```python
from build123d import *

# Parameters (mm, degrees)
SKETCH2_R           = 25
BOSS_EXTRUDE1_DEPTH = 50
BOSS_EXTRUDE2_DEPTH = 100
CIRPATTERN1_COUNT   = 3
SKETCH5_R           = 150
SKETCH5_R_2         = 90
CUT_EXTRUDE3_DEPTH  = 51
SKETCH3_R           = 6
CUT_EXTRUDE1_DEPTH  = 51


with BuildPart() as part:
    # Sketch2 → Boss-Extrude1 (new body)
    with BuildSketch(Plane(origin=(0, 0, 0), x_dir=(1, 0, 0), z_dir=(0, 1, 0))):
        Circle(SKETCH2_R)
    extrude(amount=BOSS_EXTRUDE1_DEPTH)

    # Sketch4 → Boss-Extrude2 (add)
    with BuildSketch(Plane(origin=(0, 0, 0), x_dir=(0, 0, -1), z_dir=(1, 0, 0))):
        Polygon((10, 50), (8, 50), (-10, 0), (-8, 0), align=None)
    boss_extrude2 = extrude(amount=BOSS_EXTRUDE2_DEPTH)

    # CirPattern1: Boss-Extrude2 ×3 about axis
    cirpattern1_axis = Axis((0, 0, 0), (0, 1, 0))
    for i in range(1, CIRPATTERN1_COUNT):
        add(boss_extrude2.rotate(cirpattern1_axis, i * 360 / CIRPATTERN1_COUNT))

    # Sketch5 → Cut-Extrude3 (cut, through all)
    with BuildSketch(Plane(origin=(0, 50, 0), x_dir=(1, 0, 0), z_dir=(0, 1, 0))):
        Circle(SKETCH5_R)
        Circle(SKETCH5_R_2, mode=Mode.SUBTRACT)
    extrude(amount=-CUT_EXTRUDE3_DEPTH, mode=Mode.SUBTRACT)

    # Sketch3 → Cut-Extrude1 (cut, through all)
    with BuildSketch(Plane(origin=(0, 50, 0), x_dir=(1, 0, 0), z_dir=(0, 1, 0))):
        Circle(SKETCH3_R)
    extrude(amount=-CUT_EXTRUDE1_DEPTH, mode=Mode.SUBTRACT)


solid = part.part
```
Check sheet for the modelled part. Datum: model origin and axes. Units: mm. A direction names the side the tool comes from. Round coordinates to 2 decimals unless told otherwise and drop trailing zeros. Loops run counter-clockwise (first coordinate to the right, second up) from the corner with the lowest first, then second, coordinate; pieces in that order, holes last. Notation, with made-up numbers: (-10, 52) -> (28, 52) arc R31 ccw to (28, 84) -> close; hole circle Ø8 at (19.25, -13). An arc over 180 degrees is marked (long way). Write item = value, one per line. Start each with the question number.
1) Sectioned sample at C-C, the plane y = 31. Record the cut outline in (x, z), plus the area to 3 significant figures.
2) Set-up check for faces 4 (the flat face through (-28.75, 25.35, 48.05)), 5 (the flat face through (-28.75, 24.65, -48.05)), 6 (the cylindrical face through (-45.04, 25.12, 77.92)): record each of +Z, -Z, +X, -X, +Y, -Y from which the full face is reachable in a straight line by a thin tool's end or side.
3) Sectioned sample at B-B, the plane z = 0. Record the cut outline in (x, y).
4) Thickness scan on probe 1 along Z at (x, y) = (0, 29); probe 2 along X at (y, z) = (25, 0). Record the ranges inside material, lowest first.
5) Release check for a two-part mould opening along Z. For faces 1 (the cylindrical face through (90, 25, 0)), 2 (the cylindrical face through (-25, 25, 0)), 3 (the cylindrical face through (-44.959, 25.117, -77.966)) record: released by +Z, released by -Z, zero draft, split by the parting line, or undercut.
6) Gauge pin test, flat ends, axial feed: pin 1 Ø3 at (y, z) = (22, -27) entering from +X; pin 2 Ø4 at (x, y) = (-23, 9) entering from +Z; pin 3 Ø5 at (y, z) = (14, -35.5) entering from +X. Record the tip position at first contact, or that the pin passes through.
7) Sectioned sample at D-D, the plane y = 40. Record the cut outline in (x, z), plus the area to 3 significant figures.
8) Sectioned sample at A-A, the plane x = 0. Record the cut outline in (y, z).
Results are:
q1.outline = (-47.71, -76.31) arc R90 ccw to (-46, -77.36) -> (-13.49, -21.05) arc R25 ccw to (24.8, -3.16) -> (89.94, -3.16) arc R90 ccw to (89.99, -1.16) -> (24.97, -1.16) arc R25 ccw to (-9.66, 23.06) -> (-42.24, 79.47) arc R90 ccw to (-43.99, 78.52) -> (-11.48, 22.21) arc R25 ccw to (-15.14, -19.9) -> close; hole circle Ø12 at (0, 0)
q1.area = 2,240 mm^2
q2.face_4 = -X, +Y
q2.face_5 = -X, -Y
q2.face_6 = +Z, -X, +Y, -Y
q3.outline = (-25, 0) -> (-6, 0) -> (-6, 50) -> (-25, 50) -> close; (6, 0) -> (25, 0) -> (25, 22.22) -> (90, 22.22) -> (90, 27.78) -> (25, 27.78) -> (25, 50) -> (6, 50) -> close
q4.probe_1 = -25 to -6, 6 to 25
q4.probe_2 = -25 to -6, 6 to 90
q5.face_1 = split by the parting line
q5.face_2 = undercut
q5.face_3 = released by -Z
q6.pin_1 = -12.12
q6.pin_2 = 34.07
q6.pin_3 = -12.99
q7.outline = (-50.43, -74.54) arc R90 ccw to (-48.76, -75.65) -> (-16.12, -19.11) arc R25 ccw to (24.17, -6.4) -> (89.77, -6.4) arc R90 ccw to (89.89, -4.4) -> (24.61, -4.4) arc R25 ccw to (-6.54, 24.13) -> (-39.34, 80.94) arc R90 ccw to (-41.14, 80.05) -> (-8.49, 23.51) arc R25 ccw to (-17.63, -17.73) -> close; hole circle Ø12 at (0, 0)
q7.area = 2,240 mm^2
q8.outline = (0, -25) -> (50, -25) -> (50, -6) -> (0, -6) -> close; (0, 6) -> (50, 6) -> (50, 25) -> (0, 25) -> close
